The drawing under review shows one solid part. Ordinate dimensions are in mm from its lowest x, y, z. A direction names the side the tool comes from. Give positions to 0.01 mm unless a question says otherwise; leave off trailing zeros. Write each loop counter-clockwise with the first axis right and the second up, starting at its lowest first coordinate (ties: lowest second). Pieces come first, ordered by that corner, then holes. Notation, with made-up numbers: (23, -22.5) - (36, -22.5) arc R33 ccw to (36, 15.5) - close; hole circle Ø5 at (30.5, -34). An arc over 180 degrees is marked (long way). Write item = value, one per line.
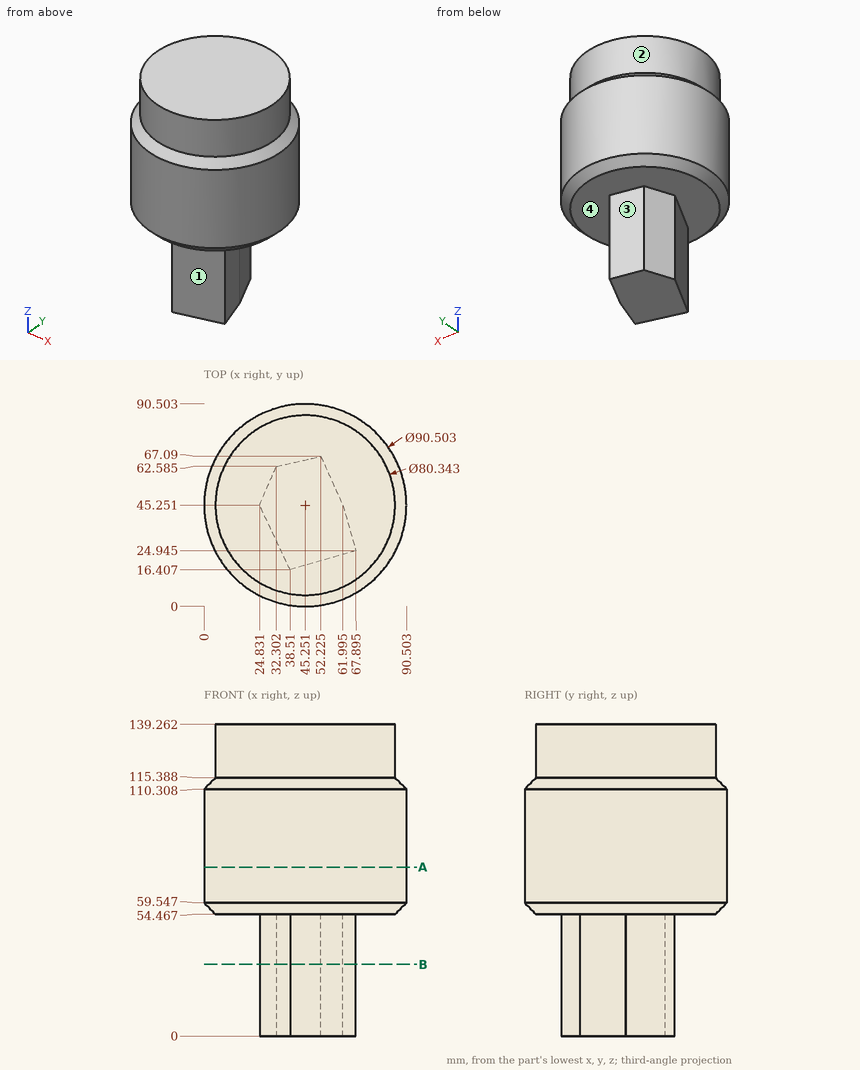
1. Take a section at A-A on z = 75.5. Give the boundary of the cut face in (x, y).
Findings below:
outline = circle Ø90.5 at (45.25, 45.25)
2. Machinability: for the marked faces 1, 2, 3 and 4, which of the approach directions +Z, -Z, +X, -X, +Y, -Y give a long, thin tool a straight path to every point of the face, cutting with its end or side? Answer none if there is none.
Findings below:
face_1 = -Z, +X, -Y
face_2 = +Z
face_3 = -Z, -X, +Y
face_4 = -Z
3. Insertion check: P1, Ø5, axis at x = 22, y = 10, coming from the -Z side; P2, Ø4, axis at x = 18.5, z = 72, coming from the -Y side; P3, Ø3, axis at y = 51.5, z = 26.5, coming from the +X side; P4, Ø8, axis at y = 41.5, z = 110.5, coming from the -X side. Each pin has a flat end and moves straight along its axis. Give the tip position at first contact, or say it passes through.
Findings below:
P1 = 54.47
P2 = 7.37
P3 = 59.87
P4 = 0
4. Take a section at B-B on z = 32. Give the boundary of the cut face in (x, y) (1 decimal).
Findings below:
outline = (24.8, 45.3) - (38.5, 16.4) - (67.9, 24.9) - (62, 45.3) - (52.2, 67.1) - (32.3, 62.6) - close
5. For line 1 (Z direction, x = 77, y = 61); line 2 (X direction, y = 44, z = 99) (1 decimal); line 3 (X direction, y = 37.5, z = 18.5), list the stretches that pass through material, from the lowest coordinate up. Write a range as from..to.
Findings below:
line_1 = 54.47..139.26
line_2 = 0..90.5
line_3 = 28.51..64.25
